The listing builds one solid part. Answer for the finished solid, in the listing's coordinates (mm). Coordinates: 2 decimals unless noted, no trailing zeros. Order: outer loops, then holes, each group sorted by start corner. A loop starts at its lowest first (then second) coordinate and runs counter-clockwise, first axis right, second up.
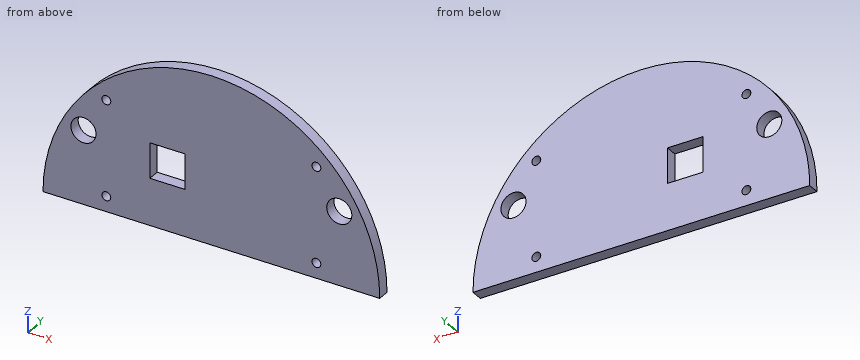
```python
from build123d import *

# Parameters (mm, degrees)
ESQUISSE1_R             = 4.25
ESQUISSE1_W             = 62.5
ESQUISSE1_H             = 25
BOSS_EXTRU_1_DEPTH      = 4
ESQUISSE2_R             = 1.5
ENL_V_MAT_EXTRU_1_DEPTH = 81.709355096
ESQUISSE3_W             = 66.086844216
ESQUISSE3_H             = 27.920410929
BOSS_EXTRU_2_DEPTH      = 4
ESQUISSE5_W             = 11.958205263
ESQUISSE5_H             = 11.958205263
ENL_V_MAT_EXTRU_2_DEPTH = 81.709355096


with BuildPart() as part:
    # Esquisse1 → Boss.-Extru.1 (new body)
    with BuildSketch(Plane(origin=(0, 0, 0), x_dir=(1, 0, 0), z_dir=(0, 1, 0))):
        with BuildLine():
            Line((-57, 0), (57, 0))
            ThreePointArc((57, 0), (0, -57), (-57, 0))
        make_face()
        with Locations(Location((-43.301270189, -25, 0), (0, 0, 270))):
            Circle(ESQUISSE1_R, mode=Mode.SUBTRACT)
        with Locations(Location((43.301270189, -25, 0), (0, 0, 270))):
            Circle(ESQUISSE1_R, mode=Mode.SUBTRACT)
        with Locations((0, -22.5)):
            Rectangle(ESQUISSE1_W, ESQUISSE1_H, mode=Mode.SUBTRACT)
    extrude(amount=BOSS_EXTRU_1_DEPTH)

    # Esquisse2 → Enlèv. mat.-Extru.1 (cut, through all)
    with BuildSketch(Plane(origin=(0, 4, 0), x_dir=(1, 0, 0), z_dir=(0, 1, 0))):
        with Locations(Location((-35.557071612, -37.554578926, 0), (0, 0, 270))):
            Circle(ESQUISSE2_R)
        with Locations(Location((-35.557071612, -5.198506408, 0), (0, 0, 270))):
            Circle(ESQUISSE2_R)
        with Locations(Location((35.557071612, -5.198506408, 0), (0, 0, 270))):
            Circle(ESQUISSE2_R)
        with Locations(Location((35.557071612, -37.554578926, 0), (0, 0, 270))):
            Circle(ESQUISSE2_R)
    extrude(amount=-ENL_V_MAT_EXTRU_1_DEPTH, mode=Mode.SUBTRACT)

    # Esquisse3 → Boss.-Extru.2 (add)
    with BuildSketch(Plane(origin=(0, 4, 0), x_dir=(1, 0, 0), z_dir=(0, 1, 0))):
        with Locations((0, -22.864687702)):
            Rectangle(ESQUISSE3_W, ESQUISSE3_H)
    extrude(amount=-BOSS_EXTRU_2_DEPTH)

    # Esquisse5 → Enlèv. mat.-Extru.2 (cut, through all)
    with BuildSketch(Plane(origin=(0, 4, 0), x_dir=(1, 0, 0), z_dir=(0, 1, 0))):
        with Locations((-14.835187955, -21.879845073)):
            Rectangle(ESQUISSE5_W, ESQUISSE5_H)
    extrude(amount=-ENL_V_MAT_EXTRU_2_DEPTH, mode=Mode.SUBTRACT)


solid = part.part
```
1) Straight lines are drawn through the part: probe 1 along Z at (x, y) = (-46, 1.6); probe 2 along X at (y, z) = (0.5, 19); probe 3 along Z at (x, y) = (47, 2.2). For each, find the intervals that lie inside material, in ascending order.
2) A cutting plane is placed at C-C, the plane y = 2.1. Write down the section's boundary in (x, z).
3) A cutting plane is placed at B-B, the plane x = 45.5. Write down the section's boundary in (y, z), plus the area to 3 significant figures.
4) Each of these flat-tipped pins is pushed along its axis until it touches: P1, Ø4, axis at x = 35.56, z = 5.2, coming from the -Y side; P2, Ø1.5, axis at y = 2, z = 26, coming from the -X side; P3, Ø2, axis at y = 3, z = 23.5, coming from the -X side; P4, Ø5, axis at x = -43.3, z = 25, coming from the +Y side. Where does it stop, or does it pass through?
5) A cutting plane is placed at A-A, the plane z = 25. Write down the section's boundary in (x, y) (3 decimals), plus the area to 3 significant figures.
6) A cutting plane is placed at D-D, the plane x = 31.5. Write down the section's boundary in (y, z), plus the area to 3 significant figures.
Working result:
1. probe 1: z = 0 to 21.72, 28.28 to 33.66
1. probe 2: x = -53.74 to -20.81, -8.86 to 53.74
1. probe 3: z = 0 to 22.91, 27.09 to 32.25
2. outline: (-57, 0) - (57, 0) arc R57 ccw to start; hole circle Ø8.5 at (-43.3, 25); hole circle Ø3 at (-35.56, 5.2); hole circle Ø3 at (-35.56, 37.55); hole (-20.81, 15.9) - (-8.86, 15.9) - (-8.86, 27.86) - (-20.81, 27.86) - close; hole circle Ø3 at (35.56, 5.2); hole circle Ø3 at (35.56, 37.55); hole circle Ø8.5 at (43.3, 25)
3. outline: (0, 0) - (4, 0) - (4, 21.36) - (0, 21.36) - close; (0, 28.64) - (4, 28.64) - (4, 34.33) - (0, 34.33) - close
3. area: 108 mm2
4. P1: stops at y = 0
4. P2: stops at x = -51.1
4. P3: stops at x = -52.37
4. P4: passes through
5. outline: (-51.225, 0) - (-47.551, 0) - (-47.551, 4) - (-51.225, 4) - close; (-39.051, 0) - (-20.814, 0) - (-20.814, 4) - (-39.051, 4) - close; (-8.856, 0) - (39.051, 0) - (39.051, 4) - (-8.856, 4) - close; (47.551, 0) - (51.225, 0) - (51.225, 4) - (47.551, 4) - close
5. area: 294 mm2
6. outline: (0, 0) - (4, 0) - (4, 47.51) - (0, 47.51) - close
6. area: 190 mm2
